```python
from build123d import *

# Parameters (mm, degrees)
SKETCH1_W           = 20
SKETCH1_H           = 20
BOSS_EXTRUDE1_DEPTH = 15
BOSS_EXTRUDE2_DEPTH = 20
CUT_EXTRUDE1_DEPTH  = 42.533119315
SKETCH4_R           = 1.905
CUT_EXTRUDE2_DEPTH  = 43.426406871
BOSS_EXTRUDE3_DEPTH = 4
BOSS_EXTRUDE4_DEPTH = 4
FILLET1_R           = 2


with BuildPart() as part:
    # Sketch1 → Boss-Extrude1 (new body)
    with BuildSketch(Plane(origin=(0, 0, 0), x_dir=(1, 0, 0), z_dir=(0, 1, 0))):
        Rectangle(SKETCH1_W, SKETCH1_H)
    extrude(amount=BOSS_EXTRUDE1_DEPTH)

    # Sketch2 → Boss-Extrude2 (add)
    with BuildSketch(Plane.XY.offset(10)):
        Polygon((10, 15), (-10, 35), (-10, 15), align=None)
        Polygon((-10, 0), (10, -20), (10, 0), align=None)
    extrude(amount=-BOSS_EXTRUDE2_DEPTH)

    # Sketch3 → Cut-Extrude1 (cut, through all)
    with BuildSketch(Plane(origin=(0, 0, -10), x_dir=(-1, 0, 0), z_dir=(0, 0, -1))):
        Polygon((-5, -15), (-5, -5), (5, -5), align=None)
    extrude(amount=-CUT_EXTRUDE1_DEPTH, mode=Mode.SUBTRACT)

    # Sketch4 → Cut-Extrude2 (cut, through all)
    with BuildSketch(Plane.XZ.offset(5)):
        Circle(SKETCH4_R)
    extrude(amount=-CUT_EXTRUDE2_DEPTH, mode=Mode.SUBTRACT)

    # Sketch5 → Boss-Extrude3 (add)
    with BuildSketch(Plane.XY.offset(10)):
        Polygon((5, -5), (5, -15), (-5, -5), align=None)
    extrude(amount=-BOSS_EXTRUDE3_DEPTH)

    # Sketch6 → Boss-Extrude4 (add)
    with BuildSketch(Plane(origin=(0, 0, -10), x_dir=(-1, 0, 0), z_dir=(0, 0, -1))):
        Polygon((5, -5), (-5, -5), (-5, -15), align=None)
    extrude(amount=-BOSS_EXTRUDE4_DEPTH)

    # Fillet1
    fillet1_edges = [part.edges().sort_by_distance(p)[0] for p in [
        (10, -20, 0),
        (0, -10, 10),
        (0, -10, -10),
        (-10, 0, 0),
    ]]
    fillet(fillet1_edges, radius=FILLET1_R)


solid = part.part
```
For this review, take the finished solid that the model builds, in its own axes (mm). A direction names the side the tool comes from. Give positions to 0.01 mm unless a question says otherwise; leave off trailing zeros. Write each loop counter-clockwise with the first axis right and the second up, starting at its lowest first coordinate (ties: lowest second). Pieces come first, ordered by that corner, then holes. Notation, with made-up numbers: M -20.5,20.25 L 3.5,20.25 A10 ccw 3.5,32.25 Z; hole C 41,-18 d5. An arc over 180 degrees is marked long. Answer as CSV lines item,"result".
1. Consider section B-B, the plane z = 0. Write out the cut boundary in (x, y) (3 decimals).
Findings:
outline,"M -10,0.828 A2 ccw -9.414,-0.586 L -5,-5 L -1.905,-5 L -1.905,26.905 L -10,35 Z; M 1.905,-5 L 5,-5 L 5,-15 L 6.586,-16.586 A2 ccw 10,-15.172 L 10,15 L 1.905,23.095 Z"
2. Consider section A-A, the plane z = 4.75. Write out the cut boundary in (x, y), then the cut area to 3 significant figures.
Findings:
outline,"M -10,0.83 A2 ccw -9.41,-0.59 L -5,-5 L 5,-5 L 5,-15 L 6.59,-16.59 A2 ccw 10,-15.17 L 10,15 L -10,35 Z"
area,"645 mm2"
3. Draft analysis for pull direction Z (two halves, no side actions). For faces 3 (the flat face through (0, 10, 10)), 4 (the cylindrical face through (-9.844, 0.053, -0.132)), 5 (the flat face through (-2.2, -5, -0.1)), state which applies: +Z half, -Z half, draft (parallel to the pull), parting line (faces both ways), or undercut.
Findings:
face 3,"+Z half"
face 4,"draft"
face 5,"undercut"
4. Consider section D-D, the plane z = 8.75. Write out the cut boundary in (x, y), then the cut area to 3 significant figures.
Findings:
outline,"M -10,0.83 A2 ccw -9.84,0.05 L 7.22,-17.01 A2 ccw 10,-15.17 L 10,15 L -10,35 Z"
area,"692 mm2"
5. For faces 1 (the flat face through (1, -9, -6)), 2 (the flat face through (0.1, 24.9, 2.4)), list the 3-axis set-ups (+Z, -Z, +X, -X, +Y, -Y) from which the entire face can be reached by the end or side of a thin tool; tool diameter is ignored.
Findings:
face 1,"-X, -Y"
face 2,"+Z, -Z, +X, +Y"
6. Wall thickness on line 1 (Z direction, x = 0, y = 7) (3 decimals); line 2 (X direction, y = -15, z = -2): over which ranges is each line inside the solid? List them lowest first.
Findings:
line 1,"z = -10 to -1.905, 1.905 to 10"
line 2,"x = 5 to 10"
7. Consider section C-C, the plane z = -7. Write out the cut boundary in (x, y), then the cut area to 3 significant figures.
Findings:
outline,"M -10,0.83 A2 ccw -9.41,-0.59 L 6.59,-16.59 A2 ccw 10,-15.17 L 10,15 L -10,35 Z"
area,"695 mm2"
8. For pin 1 (2 mm diameter, centred on x = -5, z = 3.5, fed in from -Y); pin 2 (11 mm diameter, centred on x = 1, z = -2.5, fed in from -Y); pin 3 (1 mm diameter, centred on x = 5.5, z = 2.5, fed in from -Y); pin 4 (10 mm diameter, centred on x = 5.5, z = 0, fed in from -Y), all flat-tipped, find the tip position at first contact; note any pin that passes through.
Findings:
pin 1,"stops at y = -5"
pin 2,"stops at y = -16.5"
pin 3,"stops at y = -16"
pin 4,"stops at y = -17.17"
